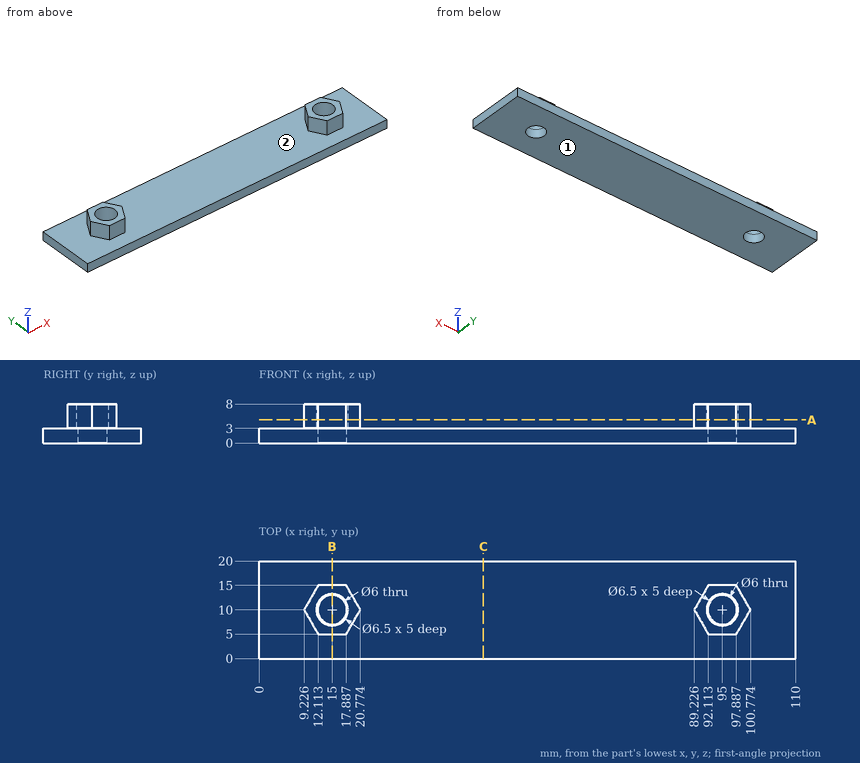
Geometry check sheet. Reference: drawing and pictorial views, mm from the part's lowest x, y, z. Give positions to 0.01 mm unless a question says otherwise; leave off trailing zeros. Order: outer loops, then holes, each group sorted by start corner. A loop starts at its lowest first (then second) coordinate and runs counter-clockwise, first axis right, second up. Notation, with made-up numbers: M 78,37 L 122,37 A25 ccw 122,63 Z; hole C -38,11 d11. An arc over 180 degrees is marked long. Answer in a Markdown table with one row per item.
1) Release check for a two-part mould opening along X. For the marked faces 1 and 2 record: +X half, -X half, draft (parallel to the pull), parting line (faces both ways), or undercut.
Filled sheet:
| item | result |
|---|---|
| face 1 | draft |
| face 2 | undercut |
2) Cross-section at B-B, the plane x = 15. Enter the section's corners in (y, z).
Filled sheet:
| item | result |
|---|---|
| outline | M 0,0 L 7,0 L 7,3 L 6.75,3 L 6.75,8 L 5,8 L 5,3 L 0,3 Z; M 13,0 L 20,0 L 20,3 L 15,3 L 15,8 L 13.25,8 L 13.25,3 L 13,3 Z |
3) Cross-section at C-C, the plane x = 46. Enter the section's corners in (y, z).
Filled sheet:
| item | result |
|---|---|
| outline | M 0,0 L 20,0 L 20,3 L 0,3 Z |
4) Cross-section at A-A, the plane z = 4.75. Enter the section's corners in (x, y), plus the area to 3 significant figures.
Filled sheet:
| item | result |
|---|---|
| outline | M 9.23,10 L 12.11,5 L 17.89,5 L 20.77,10 L 17.89,15 L 12.11,15 Z; M 89.23,10 L 92.11,5 L 97.89,5 L 100.77,10 L 97.89,15 L 92.11,15 Z; hole C 15,10 d6.5; hole C 95,10 d6.5 |
| area | 107 mm2 |
5) Gauge pin test, flat ends, axial feed: P1, Ø8, axis at x = 62.5, y = 10, coming from the +Z side; P2, Ø4, axis at x = 14.5, z = 6.5, coming from the -Y side; P3, Ø1, axis at y = 7, z = 6, coming from the +X side. Record the tip position at first contact, or that the pin passes through.
Filled sheet:
| item | result |
|---|---|
| P1 | stops at z = 3 |
| P2 | stops at y = 5 |
| P3 | stops at x = 99.33 |
6) Thickness scan on L1, parallel to Y at x = 15, z = 5.1; L2, parallel to X at y = 12.25, z = 4.5 (1 decimal); L3, parallel to X at y = 7.5, z = 3.25 (1 decimal). Record the ranges inside material, lowest first. Write a range as [from, to].
Filled sheet:
| item | result |
|---|---|
| L1 | y = [5, 6.75], [13.25, 15] |
| L2 | x = [10.5, 12.7], [17.3, 19.5], [90.5, 92.7], [97.3, 99.5] |
| L3 | x = [10.7, 12.9], [17.1, 19.3], [90.7, 92.9], [97.1, 99.3] |
